from build123d import *

# Parameters (mm, degrees)
SKETCH1_W           = 104
SKETCH1_H           = 104
BOSS_EXTRUDE1_DEPTH = 57.5
BOSS_EXTRUDE1_DRAFT = -23
SKETCH1_3_R         = 25
CUT_EXTRUDE1_DEPTH  = 94.350147295
SKETCH3_R           = 35
CUT_EXTRUDE2_DEPTH  = 10
SKETCH4_W           = 95.556530254
SKETCH4_H           = 88.466852203
CUT_EXTRUDE3_DEPTH  = 137.502747225
FILLET1_R           = 15
BOSS_EXTRUDE2_DEPTH = 10
FILLET2_R           = 5
CUT_EXTRUDE4_DEPTH  = 10


# Read off the part's stored shape, not the designer's step: Mirror2
with BuildPart() as part:
    # Sketch1 → Boss-Extrude1 (with draft: the straight prism first)
    with BuildSketch(Plane(origin=(0, 0, 0), x_dir=(1, 0, 0), z_dir=(0, 1, 0))):
        Rectangle(SKETCH1_W, SKETCH1_H)
    extrude(amount=-BOSS_EXTRUDE1_DEPTH)
    # Boss-Extrude1: the draft: its side faces are tilted about the plane it starts from
    boss_extrude1_sides = [part.faces().sort_by_distance(p)[0] for p in [
        (-52, -28.75, 0),
        (0, -28.75, 52),
        (52, -28.75, 0),
        (0, -28.75, -52),
    ]]
    draft(boss_extrude1_sides, Plane(origin=(0, 0, 0), x_dir=(1, 0, 0), z_dir=(0, 1, 0)), BOSS_EXTRUDE1_DRAFT)

    # Sketch1<3> → Cut-Extrude1 (cut, through all)
    with BuildSketch(Plane(origin=(0, 0, 0), x_dir=(1, 0, 0), z_dir=(0, 1, 0))):
        with Locations(Location((0, 0, 0), (0, 0, 270))):
            Circle(SKETCH1_3_R)
    extrude(amount=-CUT_EXTRUDE1_DEPTH, mode=Mode.SUBTRACT)

    # Sketch3 → Cut-Extrude2 (cut)
    with BuildSketch(Plane(origin=(0, 0, 0), x_dir=(1, 0, 0), z_dir=(0, 1, 0))):
        with Locations(Location((0, 0, 0), (0, 0, 270))):
            Circle(SKETCH3_R)
    extrude(amount=-CUT_EXTRUDE2_DEPTH, mode=Mode.SUBTRACT)

    # Mirror2: part across plane


with BuildPart() as part_1:
    add(part.part)
    add(part.part.mirror(Plane.ZX.offset(-57.5)))

    # Sketch4 → Cut-Extrude3 (cut, through all)
    with BuildSketch(Plane(origin=(0, 0, 0), x_dir=(1, 0, 0), z_dir=(0, 1, 0))):
        with Locations((47.778265127, 44.233426102)):
            Rectangle(SKETCH4_W, SKETCH4_H)
    extrude(amount=-CUT_EXTRUDE3_DEPTH, mode=Mode.SUBTRACT)

    # Fillet1
    fillet1_edges = [part_1.edges().sort_by_distance(p)[0] for p in [
        (-13.796349034, -57.5, -27.592698068),
        (-27.592698068, -57.5, 0),
        (0, -57.5, 27.592698068),
        (27.592698068, -57.5, 13.796349034),
    ]]
    fillet(fillet1_edges, radius=FILLET1_R)

    # Sketch5 → Boss-Extrude2 (add)
    with BuildSketch(Plane(origin=(0, 0, 0), x_dir=(1, 0, 0), z_dir=(0, 1, 0))):
        Polygon((-49, 49), (-49, -49), (49, -49), (49, -3), (49, 0), (52, 0), (52, -52), (-52, -52), (-52, 52), (0, 52), (0, 49), (-3, 49), align=None)
    extrude(amount=BOSS_EXTRUDE2_DEPTH)

    # Fillet2
    fillet2_edges = [part_1.edges().sort_by_distance(p)[0] for p in [
        (-52, 0, 0),
        (-26, 0, -52),
        (52, 0, 26),
        (0, 0, 52),
    ]]
    fillet(fillet2_edges, radius=FILLET2_R)

    # Sketch6 → Cut-Extrude4 (cut)
    with BuildSketch(Plane(origin=(0, 0, 0), x_dir=(1, 0, 0), z_dir=(0, 1, 0))):
        with BuildLine():
            Line((-42.779960262, -38.537319575), (-32.173358544, -27.930717857))
            ThreePointArc((-32.173358544, -27.930717857), (-27.930717857, -27.930717857), (-27.930717857, -32.173358544))
            Line((-27.930717857, -32.173358544), (-38.537319575, -42.779960262))
            ThreePointArc((-38.537319575, -42.779960262), (-42.779960262, -42.779960262), (-42.779960262, -38.537319575))
        make_face()
        with BuildLine():
            Line((-38.537319575, 42.779960262), (-27.930717857, 32.173358544))
            ThreePointArc((-27.930717857, 32.173358544), (-27.930717857, 27.930717857), (-32.173358544, 27.930717857))
            Line((-32.173358544, 27.930717857), (-42.779960262, 38.537319575))
            ThreePointArc((-42.779960262, 38.537319575), (-42.779960262, 42.779960262), (-38.537319575, 42.779960262))
        make_face()
        with BuildLine():
            Line((38.537319575, -42.779960262), (27.930717857, -32.173358544))
            ThreePointArc((27.930717857, -32.173358544), (27.930717857, -27.930717857), (32.173358544, -27.930717857))
            Line((32.173358544, -27.930717857), (42.779960262, -38.537319575))
            ThreePointArc((42.779960262, -38.537319575), (42.779960262, -42.779960262), (38.537319575, -42.779960262))
        make_face()
    cut_extrude4 = extrude(amount=-CUT_EXTRUDE4_DEPTH, mode=Mode.SUBTRACT)

    # Mirror3: Cut-Extrude4 across plane
    add(cut_extrude4.mirror(Plane.ZX.offset(-57.5)), mode=Mode.SUBTRACT)


solid = part_1.part
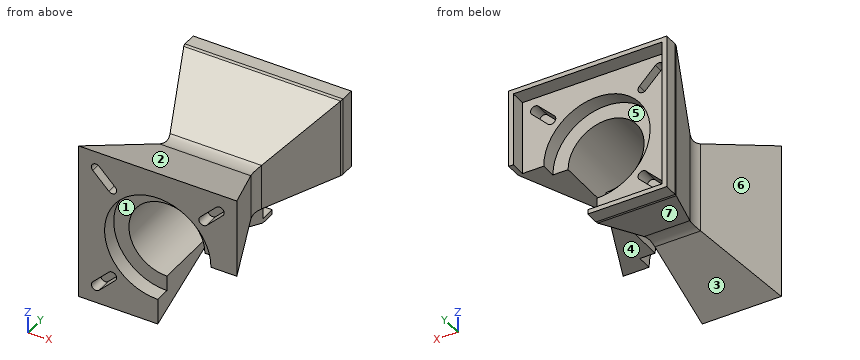
Build history of the part. All positions in model axes, mm. Face numbers are marked on the shaded views. A direction names the side the tool comes from. Round coordinates to 2 decimals unless told otherwise and drop trailing zeros. Write each loop counter-clockwise with the first axis right and the second up, starting at its lowest first coordinate (ties: lowest second). Pieces come first, ordered by that corner, then holes. Notation, with made-up numbers: M 88,55.5 L 143,55.5 A25 cw 143,87.5 Z; hole C 30,-23.5 d3. An arc over 180 degrees is marked long. Answer as a JSON object with one key per item and string values. Group by question number.
(1) Cut at A-A (x = -16.5). Give the cut face in (y, z), and give its area (3 significant figures).
(2) Cut at B-B (z = 9). Give the cut face in (x, y), and give its area (3 significant figures).
(3) Cut at D-D (x = 5). Give the cut face in (y, z).
(4) Cut at C-C (y = -7.5). Give the cut face in (x, z).
(5) Mould opens along Z. For the marked faces 1, 2 and 3 say: pulls with the +Z half, pulls with the -Z half, needs draft (parallel to the pull), parting line crosses it, or undercut.
(6) Which spindle directions (+Z, -Z, +X, -X, +Y, -Y) get a long thin tool onto all of the face, cutting with end or side? Do the marked faces 4, 5, 6 and 7. Say none if no direction does.
(7) Flat gauge pins, fed straight in: pin 1 (1.5 mm diameter, centred on x = 32.5, y = -80, fed in from -Z); pin 2 (13.5 mm diameter, centred on x = 38, z = 39.5, fed in from +Y); pin 3 (1 mm diameter, centred on y = -7, z = 3, fed in from -X). Where does each tip first touch, or does it go through?
(8) Drill centre lines: L1, parallel to X at y = 4.5, z = 39.5; L2, parallel to Y at x = -23, z = -24; L3, parallel to Y at x = -20, z = 31.5. Where is each one in solid material? Low to high.
Responses:
{
 "1": {"outline": "M -115,-52 L -63.36,-30.08 A15 cw -51.64,-30.08 L -0.94,-51.6 A5 ccw 1.02,-52 L 10,-52 L 10,-49 L 0,-49 L 0,-30.87 L -10,-30.87 L -10,-18.78 L -105,-18.78 L -105,-30.87 L -115,-30.87 Z; M -115,30.87 L -105,30.87 L -105,18.78 L -10,18.78 L -10,30.87 L 0,30.87 L 0,49 L 10,49 L 10,52 L 1.02,52 A5 ccw -0.94,51.6 L -51.64,30.08 A15 cw -63.36,30.08 L -115,52 Z", "area": "4,420 mm2"},
 "2": {"outline": "M -52,-115 L -33.82,-115 L -33.82,-105 L -23.32,-105 L -23.32,-10 L -33.82,-10 L -33.82,0 L -49,0 L -49,10 L -52,10 L -52,1.02 A5 ccw -51.6,-0.94 L -30.08,-51.64 A15 cw -30.08,-63.36 Z; M 23.32,-105 L 33.82,-105 L 33.82,-115 L 52,-115 L 30.08,-63.36 A15 cw 30.08,-51.64 L 51.6,-0.94 A5 ccw 52,1.02 L 52,10 L 49,10 L 49,0 L 33.82,0 L 33.82,-10 L 23.32,-10 Z", "area": "3,440 mm2"},
 "3": {"outline": "M -115,34.64 L -105,34.64 L -105,24.49 L -10,24.49 L -10,34.64 L 0,34.64 L 0,49 L 10,49 L 10,52 L 1.02,52 A5 ccw -0.94,51.6 L -51.64,30.08 A15 cw -63.36,30.08 L -115,52 Z"},
 "4": {"outline": "M -48.82,-48.82 L 0,-48.82 L 0,-35 A35 cw long 35,0 L 48.82,0 L 48.82,48.82 L -48.82,48.82 Z; hole M -42.78,-38.54 A3 ccw -38.54,-42.78 L -27.93,-32.17 A3 ccw -32.17,-27.93 Z; hole M -42.78,38.54 L -32.17,27.93 A3 ccw -27.93,32.17 L -38.54,42.78 A3 ccw Z; hole M 27.93,32.17 A3 ccw 32.17,27.93 L 42.78,38.54 A3 ccw 38.54,42.78 Z"},
 "5": {"face 1": "undercut", "face 2": "pulls with the +Z half", "face 3": "pulls with the -Z half"},
 "6": {"face 4": "-Z, +X, +Y, -Y", "face 5": "+Y", "face 6": "+Z, -Z, -X", "face 7": "-Z, +X, -X"},
 "7": {"pin 1": "stops at z = 0", "pin 2": "stops at y = 0", "pin 3": "stops at x = -49.24"},
 "8": {"L1": "x = -52 to -49, 49 to 52", "L2": "y = -105 to -10", "L3": "y = -115 to -66.71, -48.29 to 0"}
}
